from build123d import *

# Parameters (mm, degrees)
SKETCH1_R            = 45
JAR_BODY_DEPTH       = 120
JAR_INSIDE_START     = 120
SKETCH2_R            = 43
JAR_INSIDE_DEPTH     = 117
TURBIDITY_HOLE_START = 40
SKETCH3_W            = 27.6
SKETCH3_H            = 22.6
TURBIDITY_HOLE_DEPTH = 10


with BuildPart() as part:
    # Sketch1 → Jar_Body (new body)
    with BuildSketch(Plane(origin=(0, 0, 0), x_dir=(1, 0, 0), z_dir=(0, 1, 0))):
        with Locations(Location((0, 0, 0), (0, 0, 270))):
            Circle(SKETCH1_R)
    extrude(amount=JAR_BODY_DEPTH)

    # Sketch2 → Jar_Inside (cut)
    with BuildSketch(Plane(origin=(0, 0, 0), x_dir=(1, 0, 0), z_dir=(0, 1, 0)).offset(JAR_INSIDE_START)):
        with Locations(Location((0, 0, 0), (0, 0, 270))):
            Circle(SKETCH2_R)
    extrude(amount=-JAR_INSIDE_DEPTH, mode=Mode.SUBTRACT)

    # Sketch3 → Turbidity_Hole (cut)
    with BuildSketch(Plane(origin=(0, 0, 0), x_dir=(0, 0, -1), z_dir=(1, 0, 0)).offset(TURBIDITY_HOLE_START)):
        with Locations((0, 60)):
            Rectangle(SKETCH3_W, SKETCH3_H)
    extrude(amount=TURBIDITY_HOLE_DEPTH, mode=Mode.SUBTRACT)


solid = part.part
Can you work these out from the model? Positions are in its coordinate system, mm. A direction names the side the tool comes from. Coordinates: 2 decimals unless noted, no trailing zeros. Order: outer loops, then holes, each group sorted by start corner. A loop starts at its lowest first (then second) coordinate and runs counter-clockwise, first axis right, second up. Notation, with made-up numbers: (20.25, 20) - (55.25, 20) arc R16 ccw to (55.25, 35) - close; hole circle Ø4 at (58, 25). An arc over 180 degrees is marked (long way). Answer as a JSON object with one key per item and string values. Group by question number.
Q1. We'd pull the mould along X, two halves only. Please class faces 4 (the face through (-36.5, 120, 23.1)), 5 (the face through (-43.93, 59.16, -9.76)), 6 (the face through (-41.977, 62.319, -9.322)): +X half, -X half, draft (parallel to the pull), parting line (faces both ways), or undercut.
Q2. I need wall thicknesses on line 1 (X direction, y = 77, z = 0); line 2 (Z direction, x = 1, y = 25.5); line 3 (Z direction, x = -33, y = 95). Which ranges of each line are inside material? Lowest first, please. Write a range as from..to.
Q3. Imagine slicing it at D-D (z = 27.5). Please give me the cut outline in (x, y), and give its area (3 significant figures).
Q4. On a 3-axis mill with a long thin cutter (end or side, diameter ignored), from which of +Z, -Z, +X, -X, +Y, -Y can I reach the whole of each face in a straight line? I mean faces 1 (the face through (1, 3, -1)), 2 (the face through (43.3, 71.3, 0.2)), 3 (the face through (1, 0, -1)). Say none if no direction works.
Q5. Imagine slicing it at A-A (z = 0). Please give me the cut outline in (x, y).
Q6. Will these pins go through, and if not, where does the flat tip stop? P1, Ø0.6, axis at x = 42, y = 59.5, coming from the -Z side; P2, Ø1.5, axis at x = 10, z = 4, coming from the +Y side; P3, Ø1.5, axis at x = -24, y = 31.5, coming from the -Z side.
Q7. Imagine slicing it at B-B (x = 0). Please give me the cut outline in (y, z).
Q8. Imagine slicing it at C-C (y = 16). Please give me the cut outline in (x, z).
Determined:
{
 "1": {"face 4": "draft", "face 5": "parting line", "face 6": "undercut"},
 "2": {"line 1": "x = -45..-43, 43..45", "line 2": "z = -44.99..-42.99, 42.99..44.99", "line 3": "z = -30.59..-27.57, 27.57..30.59"},
 "3": {"outline": "(-35.62, 0) - (35.62, 0) - (35.62, 120) - (33.06, 120) - (33.06, 3) - (-33.06, 3) - (-33.06, 120) - (-35.62, 120) - close", "area": "813 mm2"},
 "4": {"face 1": "+Y", "face 2": "+X", "face 3": "+Z, -Z, +X, -X, -Y"},
 "5": {"outline": "(-45, 0) - (45, 0) - (45, 48.7) - (43, 48.7) - (43, 3) - (-43, 3) - (-43, 120) - (-45, 120) - close; (43, 71.3) - (45, 71.3) - (45, 120) - (43, 120) - close"},
 "6": {"P1": "stops at z = -16.91", "P2": "stops at y = 3", "P3": "stops at z = -38.53"},
 "7": {"outline": "(0, -45) - (120, -45) - (120, -43) - (3, -43) - (3, 43) - (120, 43) - (120, 45) - (0, 45) - close"},
 "8": {"outline": "circle Ø90 at (0, 0); hole circle Ø86 at (0, 0)"}
}
